The model under review builds one solid part; all positions refer to its coordinate system, in mm. Face numbers are marked on the shaded views. A direction names the side the tool comes from. Round coordinates to 2 decimals unless told otherwise and drop trailing zeros. Order: outer loops, then holes, each group sorted by start corner. A loop starts at its lowest first (then second) coordinate and runs counter-clockwise, first axis right, second up. Notation, with made-up numbers: (10.5, 58.25) -> (17.5, 58.25) arc R14 ccw to (17.5, 80.25) -> close; hole circle Ø5 at (79, 16.5). An arc over 180 degrees is marked (long way). Use a Markdown table: item, result. Add a question column.
```python
from build123d import *

# Parameters (mm, degrees)
SKETCH1_W           = 67.31
SKETCH1_H           = 58.42
BOSS_EXTRUDE1_DEPTH = 2.159
SKETCH2_W           = 38.862
SKETCH2_H           = 54.356
BOSS_EXTRUDE3_DEPTH = 19.05
CHAMFER1_SIZE       = 11.176


with BuildPart() as part:
    # Sketch1 → Boss-Extrude1 (new body)
    with BuildSketch(Plane(origin=(0, 0, 0), x_dir=(1, 0, 0), z_dir=(0, 1, 0))):
        Rectangle(SKETCH1_W, SKETCH1_H)
    extrude(amount=BOSS_EXTRUDE1_DEPTH)

    # Sketch2 → Boss-Extrude3 (add)
    with BuildSketch(Plane(origin=(0, 2.159, 0), x_dir=(1, 0, 0), z_dir=(0, 1, 0))):
        Rectangle(SKETCH2_W, SKETCH2_H)
    extrude(amount=BOSS_EXTRUDE3_DEPTH)

    # Sketch5 → #97 (0.275) Diameter Hole1 (revolve, cut)
    with BuildSketch(Plane(origin=(28.067, 2.159, 0), x_dir=(0, 0, 1), z_dir=(1, 0, 0))):
        Polygon((0, 0), (0, 6.162505712), (3.4925, 4.064), (3.4925, 0), align=None)
    f_97_0_275_diameter_hole1 = revolve(axis=Axis((28.067, 8.509, 0), (0, -1, 0)), mode=Mode.SUBTRACT)

    # Mirror1: #97 (0.275) Diameter Hole1 across plane
    add(f_97_0_275_diameter_hole1.mirror(Plane(origin=(0, 0, 0), x_dir=(0, 0, 1), z_dir=(1, 0, 0))), mode=Mode.SUBTRACT)

    # Chamfer1
    chamfer1_edges = [part.edges().sort_by_distance(p)[0] for p in [
        (33.655, 1.0795, 29.21),
        (-33.655, 1.0795, 29.21),
        (-33.655, 1.0795, -29.21),
        (33.655, 1.0795, -29.21),
    ]]
    chamfer(chamfer1_edges, length=CHAMFER1_SIZE)


solid = part.part
```
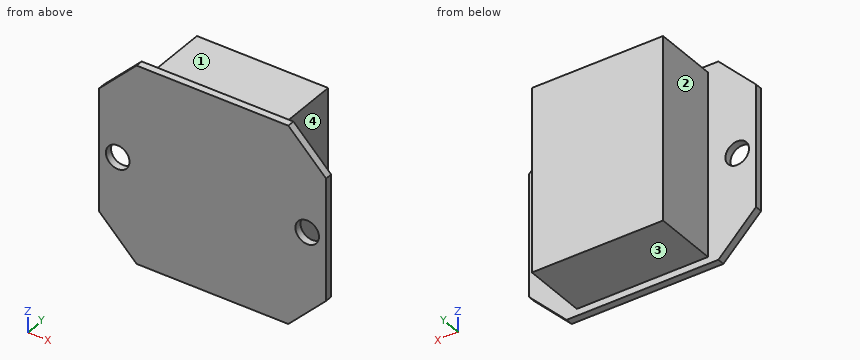
Q1. For pin 1 (4 mm diameter, centred on x = 14.5, y = 13.5, fed in from +Z); pin 2 (3 mm diameter, centred on x = 27, z = 9, fed in from +Y); pin 3 (5 mm diameter, centred on y = 10.5, z = 4, fed in from -X), all flat-tipped, find the tip position at first contact; note any pin that passes through.
Q2. For the marked faces 1, 2, 3 and 4, list the 3-axis set-ups (+Z, -Z, +X, -X, +Y, -Y) from which the entire face can be reached by the end or side of a thin tool; tool diameter is ignored.
Q3. To check wall thickness, follow line 1 along X through (y, z) = (0.9, 0) (1 decimal); line 2 along Z through (x, y) = (12, 12.75); line 3 along Y through (x, z) = (-24, 3). State the ranges of each line that lie inside material, in increasing order.
Q4. Add section D-D, the plane x = -0.5. Give the boundary of the cut face in (y, z).
Q5. Add section C-C, the plane y = 19. Give the boundary of the cut face in (x, z).
Q6. Add section B-B, the plane x = -30. Give the boundary of the cut face in (y, z), then the cut area to 3 significant figures.
Q7. Add section A-A, the plane z = 0. Give the boundary of the cut face in (x, y) (1 decimal), then the cut area to 3 significant figures.
Return value:
| question | item | result |
|---|---|---|
| 1 | pin 1 | z = 27.18 |
| 1 | pin 2 | y = 2.16 |
| 1 | pin 3 | x = -19.43 |
| 2 | face 1 | +Z, +X, -X, +Y |
| 2 | face 2 | +Z, -Z, -X, +Y |
| 2 | face 3 | -Z, +X, -X, +Y |
| 2 | face 4 | +Z, -Z, +X, +Y |
| 3 | line 1 | -33.7 to -31.6, -24.6 to 24.6, 31.6 to 33.7 |
| 3 | line 2 | -27.18 to 27.18 |
| 3 | line 3 | 0 to 2.16 |
| 4 | outline | (0, -29.21) -> (2.16, -29.21) -> (2.16, -27.18) -> (21.21, -27.18) -> (21.21, 27.18) -> (2.16, 27.18) -> (2.16, 29.21) -> (0, 29.21) -> close |
| 5 | outline | (-19.43, -27.18) -> (19.43, -27.18) -> (19.43, 27.18) -> (-19.43, 27.18) -> close |
| 6 | outline | (0, -21.69) -> (2.16, -21.69) -> (2.16, -2.91) -> (0, -2.91) -> close; (0, 2.91) -> (2.16, 2.91) -> (2.16, 21.69) -> (0, 21.69) -> close |
| 6 | area | 81.1 mm² |
| 7 | outline | (-33.7, 0) -> (-31.6, 0) -> (-31.6, 2.2) -> (-33.7, 2.2) -> close; (-24.6, 0) -> (24.6, 0) -> (24.6, 2.2) -> (19.4, 2.2) -> (19.4, 21.2) -> (-19.4, 21.2) -> (-19.4, 2.2) -> (-24.6, 2.2) -> close; (31.6, 0) -> (33.7, 0) -> (33.7, 2.2) -> (31.6, 2.2) -> close |
| 7 | area | 855 mm² |
